Could you check a few things on this drawing? It's one solid part, dimensions in mm from its lowest x, y, z. A direction names the side the tool comes from. Round coordinates to 2 decimals unless told otherwise and drop trailing zeros. Write each loop counter-clockwise with the first axis right and the second up, starting at its lowest first coordinate (ties: lowest second). Pieces come first, ordered by that corner, then holes. Notation, with made-up numbers: M 76,53.25 L 92,53.25 A11 cw 92,73.25 Z; hole C 0.25,10.5 d5. An arc over 180 degrees is marked long. One line per item, written item: value. Start each with the question number.
(1) Which directions (+Z, -Z, +X, -X, +Y, -Y) give clear straight access to the entire face, cutting with the end or side of a thin tool? Please do the marked faces 1 and 2.
(2) If I drill on L1, parallel to Y at x = 4.63, z = 15.5; L2, parallel to X at y = 51.77, z = 17.75, over which ranges is the centre line in solid material (lowest first)?
(3) I'm going to push flat-ended pins straight in: pin 1 Ø7.5 at (y, z) = (29, 8.5) entering from +X; pin 2 Ø3 at (x, y) = (11.5, 32) entering from +Z; pin 3 Ø12 at (x, z) = (45.5, 6.5) entering from +Y. Where does each tip first touch, or does it pass through?
(4) I want a section at B-B on x = 44.5. Please give me the cut outline in (y, z), and give its area (4 significant figures).
(5) I want a section at A-A on z = 13.25. Please give me the cut outline in (x, y).
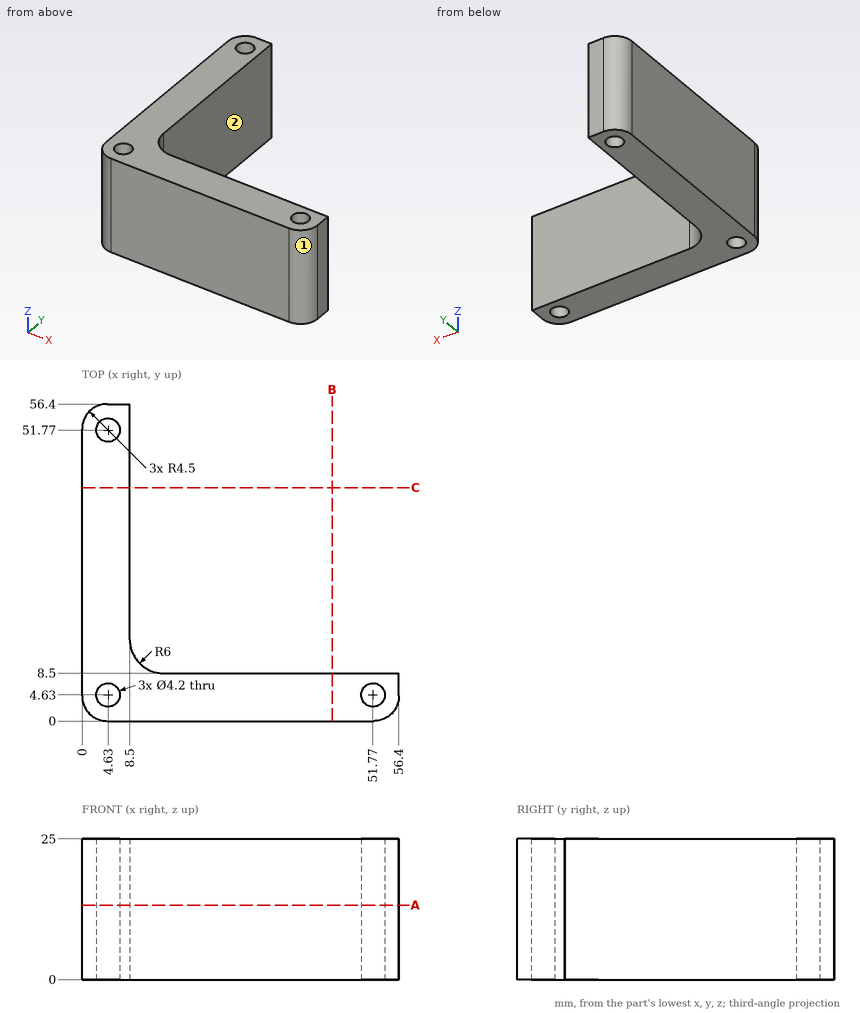
Found:
1. face 1: +Z, -Z, +X, -Y
1. face 2: +Z, -Z, +X, +Y
2. L1: y = 0 to 2.53, 6.73 to 49.67, 53.87 to 56.4
2. L2: x = 0 to 2.53, 6.73 to 8.5
3. pin 1: stops at x = 8.5
3. pin 2: passes through
3. pin 3: stops at y = 8.5
4. outline: M 0,0 L 8.5,0 L 8.5,25 L 0,25 Z
4. area: 212.5 mm²
5. outline: M 0,4.5 A4.5 ccw 4.5,0 L 51.9,0 A4.5 ccw 56.4,4.5 L 56.4,8.5 L 14.5,8.5 A6 cw 8.5,14.5 L 8.5,56.4 L 4.5,56.4 A4.5 ccw 0,51.9 Z; hole C 4.63,4.63 d4.2; hole C 4.63,51.77 d4.2; hole C 51.77,4.63 d4.2
